```python
from build123d import *

# Parameters (mm, degrees)
SKETCH1_W           = 18
SKETCH1_H           = 18
BOSS_EXTRUDE1_DEPTH = 30
FILLET1_R           = 1
SKETCH3_R           = 4
CUT_EXTRUDE1_DEPTH  = 10
SKETCH4_R           = 6
CUT_EXTRUDE2_DEPTH  = 10
SKETCH5_R           = 1.5
CUT_EXTRUDE3_DEPTH  = 19.0000001
SKETCH7_R           = 5
BOSS_EXTRUDE2_DEPTH = 4


with BuildPart() as part:
    # Sketch1 → Boss-Extrude1 (new body)
    with BuildSketch(Plane.XY):
        Rectangle(SKETCH1_W, SKETCH1_H)
    extrude(amount=-BOSS_EXTRUDE1_DEPTH)

    # Sketch2 → Cut-Revolve1 (revolve, cut)
    with BuildSketch(Plane(origin=(0, 0, 0), x_dir=(0, 0, -1), z_dir=(1, 0, 0))):
        Polygon((0, 5), (0, 12.689629666), (3.844814833, 12.689629666), align=None)
    revolve(axis=Axis((0, 0, 0), (0, 0, -1)), mode=Mode.SUBTRACT)

    # Fillet1
    fillet1_edges = [part.edges().sort_by_distance(p)[0] for p in [
        (9, -9, -15),
        (-9, -9, -15),
        (-9, 9, -15),
        (9, 9, -15),
    ]]
    fillet(fillet1_edges, radius=FILLET1_R)

    # Sketch3 → Cut-Extrude1 (cut)
    with BuildSketch(Plane.XY):
        Circle(SKETCH3_R)
    extrude(amount=-CUT_EXTRUDE1_DEPTH, mode=Mode.SUBTRACT)

    # Sketch4 → Cut-Extrude2 (cut)
    with BuildSketch(Plane(origin=(0, 0, -30), x_dir=(-1, 0, 0), z_dir=(0, 0, -1))):
        Circle(SKETCH4_R)
    extrude(amount=-CUT_EXTRUDE2_DEPTH, mode=Mode.SUBTRACT)

    # Sketch5 → Cut-Extrude3 (cut, through all)
    with BuildSketch(Plane(origin=(0, 9, 0), x_dir=(1, 0, 0), z_dir=(0, 1, 0))):
        with Locations((0, 7)):
            Circle(SKETCH5_R)
        with Locations((0, 25)):
            Circle(SKETCH5_R)
    extrude(amount=-CUT_EXTRUDE3_DEPTH, mode=Mode.SUBTRACT)

    # Sketch7 → Boss-Extrude2 (add)
    with BuildSketch(Plane.XY.offset(-14)):
        with BuildLine():
            Line((-7, 9), (7, 9))
            Line((7, 9), (7, 26))
            ThreePointArc((7, 26), (5.535533906, 29.535533906), (2, 31))
            Line((2, 31), (-2, 31))
            ThreePointArc((-2, 31), (-5.535533906, 29.535533906), (-7, 26))
            Line((-7, 26), (-7, 9))
        make_face()
        with Locations((0, 24)):
            Circle(SKETCH7_R, mode=Mode.SUBTRACT)
    extrude(amount=-BOSS_EXTRUDE2_DEPTH)


solid = part.part
```
Geometry check sheet. Reference: the model listing, model coordinates, mm. A direction names the side the tool comes from. Coordinates: 2 decimals unless noted, no trailing zeros. Write each loop counter-clockwise with the first axis right and the second up, starting at its lowest first coordinate (ties: lowest second). Pieces come first, ordered by that corner, then holes. Notation, with made-up numbers: M -12.5,-34.5 L -1.5,-34.5 A21 ccw -1.5,-18.5 Z; hole C 38.25,57 d7. An arc over 180 degrees is marked long. One line per item, written item: value. Start each with the question number.
(1) Release check for a two-part mould opening along X. For faces 6 (the face through (-8.715, -8.699, -16.946)), 7 (the face through (0, 0, -20)), 8 (the face through (8.699, -8.715, -16.946)) record: released by +X, released by -X, zero draft, split by the parting line, or undercut.
(2) Sectioned sample at C-C, the plane z = -16. Enter the section's corners in (x, y).
(3) Sectioned sample at B-B, the plane y = 24. Enter the section's corners in (x, z), and give its area (3 significant figures).
(4) Sectioned sample at D-D, the plane y = 0. Enter the section's corners in (x, z), and give its area (3 significant figures).
(5) Scan lines: line 1 along X through (y, z) = (-5, -7); line 2 along Z through (x, y) = (0, 7.45) (3 decimals); line 3 along Z through (x, y) = (0, 7.85) (3 decimals). Record each from-to range of solid material in increasing order. Write a range as [from, to].
(6) Tool access check on faces 1 (the face through (0, 18, -18)), 2 (the face through (-7, 18, -16)), 3 (the face through (0, 0, -10)), 4 (the face through (0, 18, -14)), 5 (the face through (7, 17, -16)). Record the directions out of +Z, -Z, +X, -X, +Y, -Y that give a thin tool (end or side, any length) a straight path to the whole face; none if there is none.
(7) Depth check by flat-ended pin: pin 1 (5 mm diameter, centred on x = 5, y = 22.5, fed in from +Z); pin 2 (1.2 mm diameter, centred on y = 14.5, z = -15, fed in from +X); pin 3 (8 mm diameter, centred on x = 6, z = -6, fed in from +Y). Enter the tip coordinate at first touch or a pass-through.
(8) Sectioned sample at A-A, the plane z = -7. Enter the section's corners in (x, y).
Filled sheet:
1. face 6: released by -X
1. face 7: undercut
1. face 8: released by +X
2. outline: M -9,-8 A1 ccw -8,-9 L 8,-9 A1 ccw 9,-8 L 9,8 A1 ccw 8,9 L 7,9 L 7,26 A5 ccw 2,31 L -2,31 A5 ccw -7,26 L -7,9 L -8,9 A1 ccw -9,8 Z; hole C 0,24 d10
3. outline: M -7,-18 L -5,-18 L -5,-14 L -7,-14 Z; M 5,-18 L 7,-18 L 7,-14 L 5,-14 Z
3. area: 16.0 mm²
4. outline: M -9,-30 L -6,-30 L -6,-20 L 6,-20 L 6,-30 L 9,-30 L 9,-2 L 5,0 L 4,0 L 4,-10 L -4,-10 L -4,0 L -5,0 L -9,-2 Z
4. area: 332 mm²
5. line 1: [-9, -1.5], [1.5, 9]
5. line 2: [-30, -26.5], [-23.5, -8.5], [-5.5, -1.225]
5. line 3: [-30, -26.5], [-23.5, -8.5], [-5.5, -1.425]
6. face 1: -Z, +X, -X, +Y
6. face 2: +Z, -Z, -X, +Y
6. face 3: +Z
6. face 4: +Z, +X, -X, +Y
6. face 5: +Z, -Z, +X, +Y
7. pin 1: z = -14
7. pin 2: x = 7
7. pin 3: y = 9
8. outline: M -9,-8 A1 ccw -8,-9 L -1.5,-9 L -1.5,-3.71 A4 cw -1.5,3.71 L -1.5,9 L -8,9 A1 ccw -9,8 Z; M 1.5,-9 L 8,-9 A1 ccw 9,-8 L 9,8 A1 ccw 8,9 L 1.5,9 L 1.5,3.71 A4 cw 1.5,-3.71 Z
